Autodesk Inventor part; units mm, degrees
ref_plane "YZ Plane" through (0, 0, 0) normal (1, 0, 0) x (0, 1, 0)
ref_plane "XZ Plane" through (0, 0, 0) normal (0, 1, 0) x (-1, 0, 0)
ref_plane "XY Plane" through (0, 0, 0) normal (0, 0, 1) x (1, 0, 0)
sketch "Sketch1" plane through (0, 0, 0) normal (0, 1, 0) x (-1, 0, 0)
  line L0 (0, 0) -> (127, 0)
  line L1 (127, 0) -> (127, -127)
  line L2 (127, -127) -> (0, -127)
  line L3 (0, -127) -> (0, 0)
  dimension "d0" = 127
  dimension "d1" = 127
extrude "Extrusion1" add sketch "Sketch1" along normal blind 101.6
sketch "Sketch2" plane through (0, 101.6, 0) normal (0, 1, 0) x (1, 0, 0)
  line L0 (-114.3, 114.3) -> (-12.7, 114.3)
  line L1 (-12.7, 114.3) -> (-12.7, 12.7)
  line L2 (-12.7, 12.7) -> (-114.3, 12.7)
  line L3 (-114.3, 12.7) -> (-114.3, 114.3)
  line L4 (-127, 127) -> (-127, 0)
  line L5 (0, 127) -> (-127, 127)
  point P0 (0, 0)
  dimension "d4" = 101.6
  dimension "d5" = 101.6
  dimension "d6" = 12.7
  dimension "d7" = 12.7
extrude "Extrusion2" cut sketch "Sketch2" against normal blind 76.2
sketch "Sketch3" plane through (-127, 0, 0) normal (0, 0, 1) x (1, 0, 0)
  point P0 (127, 0)
sketch "Sketch4" plane through (-127, 0, 0) normal (0, 0, 1) x (1, 0, 0)
  circle A0 centre (63.5, 76.2) radius 5.4991
  line L0 (127, 0) -> (0, 0)
  line L1 (127, 0) -> (127, 101.6)
  dimension "d10" = 10.9982
  dimension "d11" = 76.2
  dimension "d12" = 63.5
extrude "Extrusion3" cut sketch "Sketch4" against normal blind 76.2
sketch "Sketch5" plane through (-12.7, 101.6, -12.7) normal (0, 0, -1) x (-1, 0, 0)
  circle A0 centre (50.8, -25.4) radius 17.78
  line L0 (0, -76.2) -> (101.6, -76.2)
  line L1 (0, 0) -> (0, -76.2)
  point P0 (-12.7, -101.6)
  dimension "d15" = 35.56
  dimension "d16" = 50.8
  dimension "d17" = 50.8
extrude "Extrusion4" cut sketch "Sketch5" against normal blind 10.795
chamfer "Chamfer2" distance 10.795 angle 30 1 edges at (-45.72, 76.2, -12.7) measured on face at (-81.0498, 73.3479, -5.5033)
sketch "Sketch6" plane through (0, 0, 0) normal (0, -1, 0) x (1, 0, 0)
  line L0 (-57.2968, -57.2968) -> (-69.7032, -57.2968)
  line L1 (-69.7032, -57.2968) -> (-69.7032, -69.7032)
  line L2 (-69.7032, -69.7032) -> (-57.2968, -69.7032)
  line L3 (-57.2968, -69.7032) -> (-57.2968, -57.2968)
  line L4 (-127, -127) -> (0, -127)
  line L5 (0, -127) -> (0, 0)
  line L6 (0, 0) -> (-127, 0)
  line L7 (-127, 0) -> (-127, -127)
  dimension "d26" = 12.4064
  dimension "d27" = 12.4064
  dimension "d28" = 57.2968
  dimension "d29" = 57.2968
  dimension "d30" = 57.2968
  dimension "d31" = 57.2968
extrude "Extrusion5" cut sketch "Sketch6" against normal blind 25.4 contours L3 L2 L1 L0
equation "\"d6\" = -0.5 * d4 + 0.5 * d1"
equation "\"d7\" = -0.5 * d5 + 0.5 * d0"
equation "\"d12\" = 0.5 * d0"
equation "\"d28\" = -0.5 * d27 + 0.5 * d1"
equation "\"d29\" = -0.5 * d26 + 0.5 * d0"
properties part number "lampbottom"
Model file for the job. Use its own axes, mm. A direction names the side the tool comes from. Give positions to 0.01 mm unless a question says otherwise; leave off trailing zeros. Order: outer loops, then holes, each group sorted by start corner. A loop starts at its lowest first (then second) coordinate and runs counter-clockwise, first axis right, second up. Notation, with made-up numbers: M 33,48 L 91,48 A23 ccw 91,60 Z; hole C 67.5,19 d4. An arc over 180 degrees is marked long. Write item = value, one per line.
Q1. Cut at A-A, the plane x = -63.5. Count the separate pieces of the cut face and the enclosed holes in it, then the cut area to 3 significant figures.
Derived:
separate_pieces = 3
enclosed_holes = 0
area = 4,370 mm2
Q2. Drill centre lines: line 1 (X direction, y = 50.5, z = -43); line 2 (X direction, y = 76, z = -1). Where is each one in solid material? Low to high. Write a range as [from, to].
Derived:
line_1 = [-127, -114.3], [-12.7, 0]
line_2 = [-127, -69], [-58, 0]
Q3. Cut at B-B, the plane z = -105. List the corners of the cut face in (x, y).
Derived:
outline = M -127,0 L 0,0 L 0,101.6 L -12.7,101.6 L -12.7,25.4 L -114.3,25.4 L -114.3,101.6 L -127,101.6 Z
Q4. Cut at D-D, the plane x = -26.5. List the corners of the cut face in (y, z), then the cut area to 3 significant figures.
Derived:
outline = M 0,-127 L 101.6,-127 L 101.6,-114.3 L 25.4,-114.3 L 25.4,-12.7 L 101.6,-12.7 L 101.6,0 L 0,0 Z
area = 5,160 mm2
Q5. Two-plate mould, pull along Z, no slides. Class faces 4 (the flat face through (0, 50, -64)), 5 (the flat face through (-64, 64, -114.3)), 6 (the flat face through (-64, 50, -127)): pulls with the +Z half, pulls with the -Z half, needs draft (parallel to the pull), parting line crosses it, or undercut.
Derived:
face_4 = needs draft
face_5 = undercut
face_6 = pulls with the -Z half
Q6. Tool access for faces 1 (the flat face through (-64, 25.4, -76)), 2 (the conical face through (-80.284, 69.241, -2.581)), 3 (the flat face through (-63, 13, -57.297)): list every direction of +Z, -Z, +X, -X, +Y, -Y with a clear straight run to the whole face (end or side of a thin tool).
Derived:
face_1 = +Y
face_2 = none
face_3 = +Y, -Y
